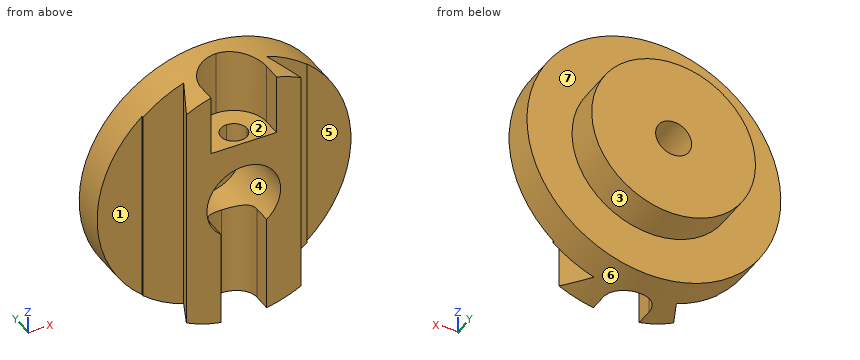
```python
from build123d import *
from build123d.topology import SkipClean

# Parameters (mm, degrees)
BOSS_EXTRUDE1_DEPTH = 77.5
SKETCH1_3_W         = 50
SKETCH1_3_H         = 22
CUT_EXTRUDE1_START  = 77.5
CUT_EXTRUDE1_DEPTH  = 39.5
CUT_EXTRUDE2_DEPTH  = 77.5
SKETCH2_OUTSIDE_W   = 202.67
SKETCH2_OUTSIDE_H   = 202.67
SKETCH2_OUTSIDE_R   = 77.5
CUT_EXTRUDE4_DEPTH  = 77.5
SKETCH4_R           = 11
CUT_EXTRUDE5_DEPTH  = 77.5
SKETCH5_R           = 22.5
CUT_EXTRUDE6_DEPTH  = 42


with BuildPart() as part:
    # Sketch1 → Boss-Extrude1 (new, symmetric)
    with SkipClean():  # the faces are left unmerged after this step: merging them gives an invalid solid
        with BuildSketch(Plane.XY):
            with BuildLine():
                Line((20, 0), (35, 0))
                Line((35, 0), (25.207539179, 21))
                Line((25.207539179, 21), (50, 21))
                Line((50, 21), (50, 22))
                Line((50, 22), (77.5, 22))
                Line((77.5, 22), (77.5, 42))
                Line((77.5, 42), (50, 42))
                Line((50, 42), (0, 42))
                Line((0, 42), (0, 31))
                ThreePointArc((0, 31), (14.142135624, 25.142135624), (20, 11))
                Line((20, 11), (20, 0))
            make_face()
            with BuildLine():
                ThreePointArc((-20, 11), (-14.142135624, 25.142135624), (0, 31))
                Line((0, 31), (0, 42))
                Line((0, 42), (-50, 42))
                Line((-50, 42), (-77.5, 42))
                Line((-77.5, 42), (-77.5, 22))
                Line((-77.5, 22), (-50, 22))
                Line((-50, 22), (-50, 21))
                Line((-50, 21), (-25.207539179, 21))
                Line((-25.207539179, 21), (-35, 0))
                Line((-35, 0), (-20, 0))
                Line((-20, 0), (-20, 11))
            make_face()
            with BuildLine():
                Line((0, 25), (0, 31))
                ThreePointArc((0, 31), (-14.142135624, 25.142135624), (-20, 11))
                Line((-20, 11), (-20, 0))
                Line((-20, 0), (-14, 0))
                Line((-14, 0), (-14, 11))
                ThreePointArc((-14, 11), (-9.899494937, 20.899494937), (0, 25))
            make_face()
            with BuildLine():
                Line((14, 0), (20, 0))
                Line((20, 0), (20, 11))
                ThreePointArc((20, 11), (14.142135624, 25.142135624), (0, 31))
                Line((0, 31), (0, 25))
                ThreePointArc((0, 25), (9.899494937, 20.899494937), (14, 11))
                Line((14, 11), (14, 0))
            make_face()
            with BuildLine():
                Line((-14, 0), (0, 0))
                Line((0, 0), (0, 3))
                ThreePointArc((0, 3), (-8, 11), (0, 19))
                Line((0, 19), (0, 25))
                ThreePointArc((0, 25), (-9.899494937, 20.899494937), (-14, 11))
                Line((-14, 11), (-14, 0))
            make_face()
            with BuildLine():
                Line((0, 0), (14, 0))
                Line((14, 0), (14, 11))
                ThreePointArc((14, 11), (9.899494937, 20.899494937), (0, 25))
                Line((0, 25), (0, 19))
                ThreePointArc((0, 19), (5.656854249, 16.656854249), (8, 11))
                ThreePointArc((8, 11), (5.656854249, 5.343145751), (0, 3))
                Line((0, 3), (0, 0))
            make_face()
        extrude(amount=BOSS_EXTRUDE1_DEPTH, both=True)

    # Sketch1_3 → Revolve1 (revolve)
    with SkipClean():  # the faces are left unmerged after this step: merging them gives an invalid solid
        with BuildSketch(Plane.XY, mode=Mode.PRIVATE) as revolve1_sk:
            with Locations((-25, 53)):
                Rectangle(SKETCH1_3_W, SKETCH1_3_H)
        revolve(revolve1_sk.sketch.rotate(Axis((0, 0, 0), (0, 1, 0)), 270), axis=Axis((0, 0, 0), (0, 1, 0)))

    # Sketch1_4 → Cut-Extrude1 (cut)
    with SkipClean():  # the faces are left unmerged after this step: merging them gives an invalid solid
        with BuildSketch(Plane.XY.offset(CUT_EXTRUDE1_START)):
            with BuildLine():
                Line((14, 0), (20, 0))
                Line((20, 0), (20, 11))
                ThreePointArc((20, 11), (14.142135624, 25.142135624), (0, 31))
                Line((0, 31), (0, 25))
                ThreePointArc((0, 25), (9.899494937, 20.899494937), (14, 11))
                Line((14, 11), (14, 0))
            make_face()
            with BuildLine():
                Line((0, 25), (0, 31))
                ThreePointArc((0, 31), (-14.142135624, 25.142135624), (-20, 11))
                Line((-20, 11), (-20, 0))
                Line((-20, 0), (-14, 0))
                Line((-14, 0), (-14, 11))
                ThreePointArc((-14, 11), (-9.899494937, 20.899494937), (0, 25))
            make_face()
            with BuildLine():
                Line((-14, 0), (0, 0))
                Line((0, 0), (0, 3))
                ThreePointArc((0, 3), (-8, 11), (0, 19))
                Line((0, 19), (0, 25))
                ThreePointArc((0, 25), (-9.899494937, 20.899494937), (-14, 11))
                Line((-14, 11), (-14, 0))
            make_face()
            with BuildLine():
                Line((0, 0), (14, 0))
                Line((14, 0), (14, 11))
                ThreePointArc((14, 11), (9.899494937, 20.899494937), (0, 25))
                Line((0, 25), (0, 19))
                ThreePointArc((0, 19), (5.656854249, 16.656854249), (8, 11))
                ThreePointArc((8, 11), (5.656854249, 5.343145751), (0, 3))
                Line((0, 3), (0, 0))
            make_face()
        extrude(amount=-CUT_EXTRUDE1_DEPTH, mode=Mode.SUBTRACT)

    # Sketch1_5 → Cut-Extrude2 (cut)
    with BuildSketch(Plane.XY):
        with BuildLine():
            Line((-14, 0), (0, 0))
            Line((0, 0), (0, 3))
            ThreePointArc((0, 3), (-8, 11), (0, 19))
            Line((0, 19), (0, 25))
            ThreePointArc((0, 25), (-9.899494937, 20.899494937), (-14, 11))
            Line((-14, 11), (-14, 0))
        make_face()
        with BuildLine():
            Line((0, 0), (14, 0))
            Line((14, 0), (14, 11))
            ThreePointArc((14, 11), (9.899494937, 20.899494937), (0, 25))
            Line((0, 25), (0, 19))
            ThreePointArc((0, 19), (5.656854249, 16.656854249), (8, 11))
            ThreePointArc((8, 11), (5.656854249, 5.343145751), (0, 3))
            Line((0, 3), (0, 0))
        make_face()
    extrude(amount=-CUT_EXTRUDE2_DEPTH, mode=Mode.SUBTRACT)

    # Sketch2 outside → Cut-Extrude4 (cut)
    with BuildSketch(Plane(origin=(0, 64, 0), x_dir=(1, 0, 0), z_dir=(0, 1, 0))):
        Rectangle(SKETCH2_OUTSIDE_W, SKETCH2_OUTSIDE_H)
        with Locations(Location((0, 0, 0), (0, 0, 270))):
            Circle(SKETCH2_OUTSIDE_R, mode=Mode.SUBTRACT)
    extrude(amount=-CUT_EXTRUDE4_DEPTH, mode=Mode.SUBTRACT)

    # Sketch4 → Cut-Extrude5 (cut)
    with BuildSketch(Plane(origin=(0, 64, 0), x_dir=(1, 0, 0), z_dir=(0, 1, 0))):
        with Locations(Location((0, 0, 0), (0, 0, 270))):
            Circle(SKETCH4_R)
    extrude(amount=-CUT_EXTRUDE5_DEPTH, mode=Mode.SUBTRACT)

    # Sketch5 → Cut-Extrude6 (cut)
    with BuildSketch(Plane.XZ):
        Circle(SKETCH5_R)
    extrude(amount=-CUT_EXTRUDE6_DEPTH, mode=Mode.SUBTRACT)


solid = part.part
```
Build history of the part. All positions in model axes, mm. Face numbers are marked on the shaded views. A direction names the side the tool comes from. Coordinates: 2 decimals unless noted, no trailing zeros. Write each loop counter-clockwise with the first axis right and the second up, starting at its lowest first coordinate (ties: lowest second). Pieces come first, ordered by that corner, then holes.
1. Pull direction Z, two halves, no side cores. Call the marked faces 1, 2, 3 and 4: released by +Z, released by -Z, zero draft, split by the parting line, or undercut.
Answer block:
face 1: zero draft
face 2: released by +Z
face 3: split by the parting line
face 4: undercut
2. Band-saw the part on B-B, the plane y = 55. Give the cut face in (x, z).
Answer block:
outline: circle Ø100 at (0, 0); hole circle Ø22 at (0, 0)
3. Drill centre lines: probe 1 along X at (y, z) = (50.25, 0); probe 2 along Y at (x, z) = (35.5, -37.5); probe 3 along Y at (x, z) = (-39, -21). Where is each one in solid material? Low to high.
Answer block:
probe 1: x = -50 to -11, 11 to 50
probe 2: y = 21 to 42
probe 3: y = 21 to 64
4. Drop flat-ended pins along their axis: pin 1 (6 mm diameter, centred on y = 42, z = 6, fed in from +X); pin 2 (1 mm diameter, centred on x = -15.5, z = -10.5, fed in from -Y); pin 3 (6 mm diameter, centred on y = 23, z = 15, fed in from -X). Give the stop position or say it passes through.
Answer block:
pin 1: stops at x = 77.44
pin 2: stops at y = 42
pin 3: stops at x = -76.57
5. 3-axis set-ups, long thin cutter, end or side, ignore diameter. For the marked faces 5, 6 and 7: which of +Z, -Z, +X, -X, +Y, -Y reach the whole face in a straight line?
Answer block:
face 5: +Z, -Z, +X, -Y
face 6: +Y, -Y
face 7: +Y
6. Band-saw the part on D-D, the plane z = 17. Give the cut face in (x, y), and give its area (3 significant figures).
Answer block:
outline: (-75.61, 22) - (-50, 22) - (-50, 21) - (-25.21, 21) - (-35, 0) - (-14.74, 0) - (-14.74, 42) - (14.74, 42) - (14.74, 0) - (35, 0) - (25.21, 21) - (50, 21) - (50, 22) - (75.61, 22) - (75.61, 42) - (47.02, 42) - (47.02, 64) - (-47.02, 64) - (-47.02, 42) - (-75.61, 42) - close
area: 5,220 mm2
7. Band-saw the part on A-A, the plane z = 0. Give the cut face in (x, y), and give its area (3 significant figures).
Answer block:
outline: (-77.5, 22) - (-50, 22) - (-50, 21) - (-25.21, 21) - (-35, 0) - (-22.5, 0) - (-22.5, 42) - (-11, 42) - (-11, 64) - (-50, 64) - (-50, 42) - (-77.5, 42) - close; (11, 42) - (22.5, 42) - (22.5, 0) - (35, 0) - (25.21, 21) - (50, 21) - (50, 22) - (77.5, 22) - (77.5, 42) - (50, 42) - (50, 64) - (11, 64) - close
area: 4,290 mm2
8. Band-saw the part on C-C, the plane x = -62. Give the cut face in (y, z), and give its area (3 significant figures).
Answer block:
outline: (22, -46.5) - (42, -46.5) - (42, 46.5) - (22, 46.5) - close
area: 1,860 mm2
